Read the model definition and answer for the solid it produces. Units are mm, in the model's axes. A direction names the side the tool comes from. Coordinates: 2 decimals unless noted, no trailing zeros. Write each loop counter-clockwise with the first axis right and the second up, starting at its lowest first coordinate (ties: lowest second). Pieces come first, ordered by that corner, then holes.
(1) Section C-C on y = 4.75 is taken. Write down the section's boundary in (x, z).
(2) Which of the six approach directions +Z, -Z, +X, -X, +Y, -Y give full straight-line access (tool end or side, diameter ignored) to faces 1 (the flat face through (0, 6.2, 0)), 2 (the flat face through (3, 5, 0)), 3 (the flat face through (5, 0, 2))?
(3) Section D-D on y = 1.75 is taken. Write down the section's boundary in (x, z), then the cut area to 3 significant figures.
(4) The mould has two halves that part along X. Classify faces 4 (the flat face through (6.5, 6.2, 0)), 5 (the cylindrical face through (6.7, 6.5, -0.1)), 6 (the flat face through (-0.5, 3, 0)): +X half, -X half, draft (parallel to the pull), parting line (faces both ways), or undercut.
(5) Find the intervals of material crossed by probe 1 along X at (y, z) = (3.85, 0); probe 2 along Z at (x, y) = (4.75, 2.5); probe 3 along Z at (x, y) = (3, 1), in increasing order.
(6) Section B-B on x = 3.25 is taken. Write down the section's boundary in (y, z).
(7) Section A-A on z = 0 is taken. Write down the section's boundary in (x, y).
(8) Given pin 1 (2 mm diameter, centred on x = 6, y = 3.5, fed in from +Z); pin 2 (1.1 mm diameter, centred on x = 2.5, z = -0.5, fed in from -Y); pin 3 (3 mm diameter, centred on x = 3.25, z = 0, fed in from +Y), each flat-ended and moving along its own axis, determine where each tip first touches the part or whether it passes through.
from build123d import *

# Parameters (mm, degrees)
BOSS_EXTRUDE1_DEPTH = 6.5
BOSS_EXTRUDE2_DEPTH = 0.5
SKETCH4_R           = 1.9
CUT_EXTRUDE1_DEPTH  = 5


with BuildPart() as part:
    # Sketch2 → Boss-Extrude1 (new body)
    with BuildSketch(Plane(origin=(0, 0, 0), x_dir=(0, 0, -1), z_dir=(1, 0, 0))):
        with BuildLine():
            Line((-6, 0), (6, 0))
            ThreePointArc((6, 0), (0, 6), (-6, 0))
        make_face()
    extrude(amount=BOSS_EXTRUDE1_DEPTH)

    # Sketch3 → Boss-Extrude2 (add)
    with BuildSketch(Plane(origin=(6.5, 0, 0), x_dir=(0, 0, -1), z_dir=(1, 0, 0))):
        with BuildLine():
            Line((-6.5, 0), (6.5, 0))
            ThreePointArc((6.5, 0), (0, 6.5), (-6.5, 0))
        make_face()
    boss_extrude2 = extrude(amount=BOSS_EXTRUDE2_DEPTH)

    # Mirror1: Boss-Extrude2 across plane
    add(boss_extrude2.mirror(Plane(origin=(3.25, 0, 0), x_dir=(0, 0, 1), z_dir=(1, 0, 0))))

    # Sketch4 → Cut-Extrude1 (cut)
    with BuildSketch(Plane.XZ):
        with Locations(Location((3.25, 0, 0), (0, 0, 270))):
            Circle(SKETCH4_R)
    extrude(amount=-CUT_EXTRUDE1_DEPTH, mode=Mode.SUBTRACT)


solid = part.part
Response:
1. outline: (-0.5, -4.44) - (0, -4.44) - (0, -3.67) - (6.5, -3.67) - (6.5, -4.44) - (7, -4.44) - (7, 4.44) - (6.5, 4.44) - (6.5, 3.67) - (0, 3.67) - (0, 4.44) - (-0.5, 4.44) - close; hole circle Ø3.8 at (3.25, 0)
2. face 1: +Y
2. face 2: -Y
2. face 3: +Z, -Z, +X, -X, -Y
3. outline: (-0.5, -6.26) - (0, -6.26) - (0, -5.74) - (6.5, -5.74) - (6.5, -6.26) - (7, -6.26) - (7, 6.26) - (6.5, 6.26) - (6.5, 5.74) - (0, 5.74) - (0, 6.26) - (-0.5, 6.26) - close; hole circle Ø3.8 at (3.25, 0)
3. area: 75.8 mm2
4. face 4: undercut
4. face 5: draft
4. face 6: -X half
5. probe 1: x = -0.5 to 1.35, 5.15 to 7
5. probe 2: z = -5.45 to -1.17, 1.17 to 5.45
5. probe 3: z = -5.92 to -1.88, 1.88 to 5.92
6. outline: (0, -6) arc R6 ccw to (0, 6) - (0, 1.9) - (5, 1.9) - (5, -1.9) - (0, -1.9) - close
7. outline: (-0.5, 0) - (1.35, 0) - (1.35, 5) - (5.15, 5) - (5.15, 0) - (7, 0) - (7, 6.5) - (6.5, 6.5) - (6.5, 6) - (0, 6) - (0, 6.5) - (-0.5, 6.5) - close
8. pin 1: stops at z = 5.94
8. pin 2: stops at y = 5
8. pin 3: stops at y = 6
